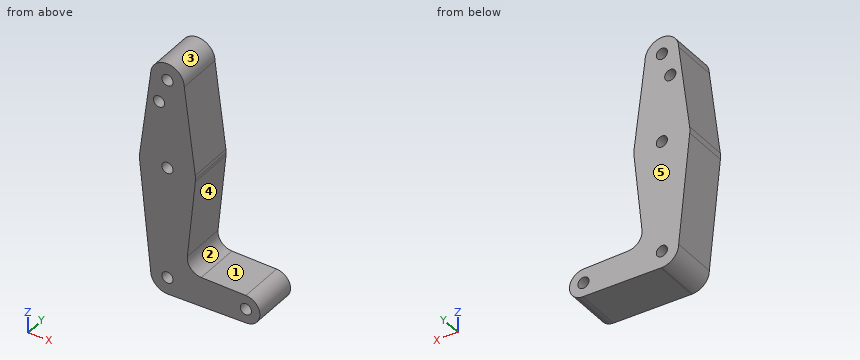
```python
from build123d import *

# Parameters (mm, degrees)
F0_R     = 3.175
F1_DEPTH = 25.4


# Not quite as in the source:
# - ends of sketch curves that miss each other by under 0.0002 mm in the source are joined


with BuildPart() as f1:
    # F0 (on Front) → F1 (new body)
    with BuildSketch(Plane.XZ):
        with BuildLine():
            ThreePointArc((9.525, 114.3), (0, 123.825), (-9.525, 114.3))
            ThreePointArc((-9.525, 114.3), (0, 104.775), (9.525, 114.3))
        make_face()
        with Locations((0, 114.3)):
            Circle(F0_R, mode=Mode.SUBTRACT)
        with BuildLine():
            Line((-9.525, 114.3), (-15.7474569047, 65.5082893304))
            ThreePointArc((-15.7474569047, 65.5082893304), (0, 79.375), (15.7474569047, 65.5082893304))
            Line((15.7474569047, 65.5082893304), (9.525, 114.3))
            ThreePointArc((9.525, 114.3), (0, 104.775), (-9.525, 114.3))
        make_face()
        with Locations((-4.7625, 100.0252)):
            Circle(F0_R, mode=Mode.SUBTRACT)
        with BuildLine():
            ThreePointArc((-9.525, 0), (0, 9.525), (9.525, 0))
            ThreePointArc((9.525, 0), (6.9705567315, -6.4912990883), (0.6773435479, -9.500885786))
            Line((0.6773435479, -9.500885786), (44.7324052746, -7.9324746146))
            ThreePointArc((44.7324052746, -7.9324746146), (36.5137564458, -0.1412249921), (44.45, 7.9375))
            Line((44.45, 7.9375), (19.160010759, 7.9375))
            ThreePointArc((19.160010759, 7.9375), (13.2639846378, 10.5545437096), (11.2496616365, 16.68272))
            Line((11.2496616365, 16.68272), (15.7954255641, 61.9125))
            ThreePointArc((15.7954255641, 61.9125), (15.8550939106, 62.7052534459), (15.875, 63.5))
            ThreePointArc((15.875, 63.5), (15.8430821396, 64.5061676396), (15.7474569047, 65.5082893304))
            ThreePointArc((15.7474569047, 65.5082893304), (0, 79.375), (-15.7474569047, 65.5082893304))
            ThreePointArc((-15.7474569047, 65.5082893304), (-15.8735876139, 63.7117575563), (-15.795425611, 61.9125004674))
            Line((-15.795425611, 61.9125004674), (-9.525, 0))
        make_face()
        with Locations((0, 63.5)):
            Circle(F0_R, mode=Mode.SUBTRACT)
        with BuildLine():
            ThreePointArc((0.6773435479, -9.500885786), (6.9705567315, -6.4912990883), (9.525, 0))
            ThreePointArc((9.525, 0), (0, 9.525), (-9.525, 0))
            ThreePointArc((-9.525, 0), (-6.7351920908, -6.7351920908), (0, -9.525))
            Line((0, -9.525), (0.6773435479, -9.500885786))
        make_face()
        Circle(F0_R, mode=Mode.SUBTRACT)
        with BuildLine():
            ThreePointArc((44.45, 7.9375), (36.5137564458, -0.1412249921), (44.7324052746, -7.9324746146))
            ThreePointArc((44.7324052746, -7.9324746146), (50.1616327839, -5.5119104847), (52.3875, 0))
            ThreePointArc((52.3875, 0), (50.0626600757, 5.6126600757), (44.45, 7.9375))
        make_face()
        with Locations((44.45, 0)):
            Circle(F0_R, mode=Mode.SUBTRACT)
    extrude(amount=F1_DEPTH)


solid = f1.part
```
For this review, take the finished solid that the model builds, in its own axes (mm). Face numbers are marked on the shaded views. A direction names the side the tool comes from. Round coordinates to 2 decimals unless told otherwise and drop trailing zeros. Order: outer loops, then holes, each group sorted by start corner. A loop starts at its lowest first (then second) coordinate and runs counter-clockwise, first axis right, second up. Notation, with made-up numbers: (35, 23.25) -> (39, 23.25) arc R12 ccw to (39, 43.25) -> close; hole circle Ø5 at (9.5, 8). An arc over 180 degrees is marked (long way). Use a Markdown table: item, result.
Item 1: For line 1 along Z through (x, y) = (0, -20) (3 decimals); line 2 along X through (y, z) = (-10, 114); line 3 along Z through (x, y) = (27.5, -14.75), list the stretches that pass through material, from the lowest coordinate up. Write a range as [from, to].
Resolved:
| item | result |
|---|---|
| line 1 | z = [-9.525, -3.175], [3.175, 60.325], [66.675, 111.125], [117.475, 123.825] |
| line 2 | x = [-9.56, -3.16], [3.16, 9.56] |
| line 3 | z = [-8.55, 7.94] |
Item 2: Take a section at C-C (z = 26.5). State the section outline as (x, y) points.
Resolved:
| item | result |
|---|---|
| outline | (-12.21, -25.4) -> (12.24, -25.4) -> (12.24, 0) -> (-12.21, 0) -> close |
Item 3: Take a section at B-B (x = 37.5). State the section outline as (y, z) points, plus the area to 3 significant figures.
Resolved:
| item | result |
|---|---|
| outline | (-25.4, -8.19) -> (0, -8.19) -> (0, 7.94) -> (-25.4, 7.94) -> close |
| area | 410 mm² |
Item 4: For pin 1 (7.5 mm diameter, centred on x = 35, y = -16, fed in from +Z); pin 2 (8.5 mm diameter, centred on x = 0, z = 63.5, fed in from +Y); pin 3 (5.5 mm diameter, centred on x = 0, z = 114.3, fed in from -Y); pin 4 (1 mm diameter, centred on y = -7, z = 37.5, fed in from +X), all flat-tipped, find the tip position at first contact; note any pin that passes through.
Resolved:
| item | result |
|---|---|
| pin 1 | stops at z = 7.94 |
| pin 2 | stops at y = 0 |
| pin 3 | passes through |
| pin 4 | stops at x = 13.39 |
Item 5: Machinability: for the marked faces 1 and 2, which of the approach directions +Z, -Z, +X, -X, +Y, -Y give a long, thin tool a straight path to every point of the face, cutting with its end or side? Answer none if there is none.
Resolved:
| item | result |
|---|---|
| face 1 | +Z, +X, +Y, -Y |
| face 2 | +X, +Y, -Y |
Item 6: Take a section at A-A (y = -6.75). State how many separate pieces and enclosed holes the cut face has, plus the area to 3 significant figures.
Resolved:
| item | result |
|---|---|
| separate pieces | 1 |
| enclosed holes | 5 |
| area | 3,750 mm² |
Item 7: Draft analysis for pull direction Z (two halves, no side actions). For the marked faces 3, 4 and 5, state which applies: +Z half, -Z half, draft (parallel to the pull), parting line (faces both ways), or undercut.
Resolved:
| item | result |
|---|---|
| face 3 | +Z half |
| face 4 | undercut |
| face 5 | draft |
